CAD build for the part. Positions are in the model's coordinates, mm. Give positions to 0.01 mm unless a question says otherwise; leave off trailing zeros. Write each loop counter-clockwise with the first axis right and the second up, starting at its lowest first coordinate (ties: lowest second). Pieces come first, ordered by that corner, then holes. Notation, with made-up numbers: M 6.25,4 L 52.25,4 A14 cw 52.25,25 Z; hole C 17,63.25 d10. An arc over 180 degrees is marked long. One line per question, with ' | ' between items. Start each with the question number.
1. Wall check: L1, parallel to Z at x = 63.5, y = 0.2; L2, parallel to X at y = 0.35, z = 3; L3, parallel to X at y = 1.95, z = -12. Give the ranges that are in metal, low to high.
2. Cut at B-B, the plane z = -1.5. Write the cut outline in (x, y), then the cut area to 3 significant figures.
3. Cut at D-D, the plane y = 0.7. Write the cut outline in (x, z), then the cut area to 3 significant figures.
4. Cut at A-A, the plane x = 79.5. Write the cut outline in (y, z), then the cut area to 3 significant figures.
5. Cut at C-C, the plane x = -21. Write the cut outline in (y, z).
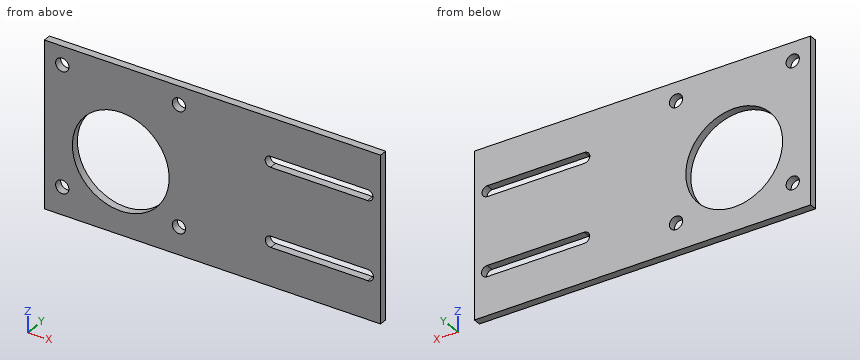
```python
from build123d import *

# Parameters (mm, degrees)
SKETCH1_W           = 132
SKETCH1_H           = 65
BOSS_EXTRUDE1_DEPTH = 3
SKETCH2_R           = 19
SKETCH2_R_2         = 2.6
CUT_EXTRUDE3_DEPTH  = 3
CUT_EXTRUDE5_DEPTH  = 3


with BuildPart() as part:
    # Sketch1 → Boss-Extrude1 (new body)
    with BuildSketch(Plane(origin=(0, 0, 0), x_dir=(1, 0, 0), z_dir=(0, 1, 0))):
        with Locations((27.886363636, -7.829545455)):
            Rectangle(SKETCH1_W, SKETCH1_H)
    extrude(amount=BOSS_EXTRUDE1_DEPTH)

    # Sketch2 → Cut-Extrude3 (cut)
    with BuildSketch(Plane(origin=(0, 3, 0), x_dir=(1, 0, 0), z_dir=(0, 1, 0))):
        with Locations(Location((-8.113636364, -3.555015025, 0), (0, 0, 270))):
            Circle(SKETCH2_R)
        with Locations(Location((-31.076450467, 13.876917129, 0), (0, 0, 270))):
            Circle(SKETCH2_R_2)
        with Locations(Location((-31.076450467, -33.123082871, 0), (0, 0, 270))):
            Circle(SKETCH2_R_2)
        with Locations(Location((14.725739937, 13.876917129, 0), (0, 0, 270))):
            Circle(SKETCH2_R_2)
        with Locations(Location((14.725739937, -33.123082871, 0), (0, 0, 270))):
            Circle(SKETCH2_R_2)
    extrude(amount=-CUT_EXTRUDE3_DEPTH, mode=Mode.SUBTRACT)

    # Sketch5 → Cut-Extrude5 (cut)
    with BuildSketch(Plane(origin=(0, 3, 0), x_dir=(1, 0, 0), z_dir=(0, 1, 0))):
        with BuildLine():
            Line((50.793786384, 9.670454545), (88.893786384, 9.670454545))
            ThreePointArc((88.893786384, 9.670454545), (91.052786384, 7.511454545), (88.893786384, 5.352454545))
            Line((88.893786384, 5.352454545), (50.793786384, 5.352454545))
            ThreePointArc((50.793786384, 5.352454545), (48.634786384, 7.511454545), (50.793786384, 9.670454545))
        make_face()
        with BuildLine():
            Line((50.658524024, -21.129545455), (88.758524024, -21.129545455))
            ThreePointArc((88.758524024, -21.129545455), (90.858524024, -23.229545455), (88.758524024, -25.329545455))
            Line((88.758524024, -25.329545455), (50.658524024, -25.329545455))
            ThreePointArc((50.658524024, -25.329545455), (48.558524024, -23.229545455), (50.658524024, -21.129545455))
        make_face()
    extrude(amount=-CUT_EXTRUDE5_DEPTH, mode=Mode.SUBTRACT)


solid = part.part
```
Here are the results:
1) L1: -24.67 to -9.67, -5.35 to 21.13, 25.33 to 40.33 | L2: -38.11 to -27.11, 10.88 to 93.89 | L3: -38.11 to -32.88, -29.28 to -19.02, 2.8 to 12.93, 16.52 to 93.89
2) outline: M -38.11,0 L -26.43,0 L -26.43,3 L -38.11,3 Z; M 10.2,0 L 93.89,0 L 93.89,3 L 10.2,3 Z | area: 286 mm^2
3) outline: M -38.11,-24.67 L 93.89,-24.67 L 93.89,40.33 L -38.11,40.33 Z; hole C -31.08,-13.88 d5.2; hole C -31.08,33.12 d5.2; hole C -8.11,3.56 d38; hole C 14.73,-13.88 d5.2; hole C 14.73,33.12 d5.2; hole M 50.66,21.13 L 88.76,21.13 A2.1 ccw 88.76,25.33 L 50.66,25.33 A2.1 ccw Z; hole M 50.79,-9.67 L 88.89,-9.67 A2.16 ccw 88.89,-5.35 L 50.79,-5.35 A2.16 ccw Z | area: 7,010 mm^2
4) outline: M 0,-24.67 L 3,-24.67 L 3,-9.67 L 0,-9.67 Z; M 0,-5.35 L 3,-5.35 L 3,21.13 L 0,21.13 Z; M 0,25.33 L 3,25.33 L 3,40.33 L 0,40.33 Z | area: 169 mm^2
5) outline: M 0,-24.67 L 3,-24.67 L 3,-10.41 L 0,-10.41 Z; M 0,17.52 L 3,17.52 L 3,40.33 L 0,40.33 Z
